The listing builds one solid part. Answer for the finished solid, in the listing's coordinates (mm). Coordinates: 2 decimals unless noted, no trailing zeros. Order: outer loops, then holes, each group sorted by start corner. A loop starts at its lowest first (then second) coordinate and runs counter-clockwise, first axis right, second up. Notation, with made-up numbers: (-33, 18.5) -> (-21, 18.5) arc R12 cw to (-21, 28.5) -> close; hole circle Ø4 at (-16, 78.25). An arc over 180 degrees is marked (long way). Answer in a Markdown table with one row per item. Add a question column.
```python
from build123d import *

# Parameters (mm, degrees)
BOSS_EXTRUDE1_DEPTH = 3


with BuildPart() as part:
    # Sketch3 → Boss-Extrude1 (new body)
    with BuildSketch(Plane.XY):
        with BuildLine():
            ThreePointArc((-21.06925633, 1.560185503), (-21.702383426, -4.120337722), (-16.861546239, -7.159332517))
            Line((-16.861546239, -7.159332517), (-16.235942246, -7.122800897))
            ThreePointArc((-16.235942246, -7.122800897), (-14.247317716, -6.480760333), (-12.653836147, -5.128850538))
            ThreePointArc((-12.653836147, -5.128850538), (21.262556938, 11.81913919), (56.062735888, -3.230898045))
            ThreePointArc((56.062735888, -3.230898045), (59.548283557, -3.823314658), (60.140700171, -0.337766989))
            ThreePointArc((60.140700171, -0.337766989), (19.96998669, 19.192613792), (-21.06925633, 1.560185503))
        make_face()
        Polygon((-14.842971244, -1.436629161), (-14.495267888, -1.784332517), (-14.848821278, -2.137885908), (-14.637840313, -2.550832882), (-15.083092963, -2.778319315), (-15.00954079, -3.236171091), (-15.503211236, -3.315477399), (-15.574237606, -3.773727796), (-16.068337858, -3.697144889), (-16.277038544, -4.111248976), (-16.723538831, -3.886221213), (-17.049626765, -4.215925369), (-17.405124343, -3.864326917), (-17.816901648, -4.077581746), (-18.046839834, -3.633590269), (-18.504279068, -3.70966601), (-18.586306367, -3.21644038), (-19.04494145, -3.147941973), (-18.971084274, -2.65342694), (-19.386332882, -2.447012878), (-19.163770631, -1.999278532), (-19.495267888, -1.67501361), (-19.145635065, -1.317582653), (-19.361157273, -0.906987537), (-18.918440472, -0.674604591), (-18.997037466, -0.217591808), (-18.504271649, -0.132846012), (-18.438303288, 0.326159812), (-17.94338851, 0.255030612), (-17.73926735, 0.671411115), (-17.290312559, 0.451321143), (-16.967880508, 0.784601421), (-16.60852704, 0.436944858), (-16.199126599, 0.654727893), (-15.964305958, 0.213299227), (-15.507733522, 0.294415085), (-15.420271807, -0.197875935), (-14.960909199, -0.261312244), (-15.029308259, -0.756611718), (-14.611808522, -0.958433771), align=None, mode=Mode.SUBTRACT)
    extrude(amount=BOSS_EXTRUDE1_DEPTH)


solid = part.part
```
Q1. Determine the mould class of faces 1 (the face through (20.7, 11.8, 1.5)), 2 (the face through (59.503, -3.855, 1.479)), 3 (the face through (-21.74, -4.04, 1.48)), 4 (the face through (-14.273, -6.495, 1.479)) for opening direction X: +X half, -X half, draft (parallel to the pull), parting line (faces both ways), or undercut.
Q2. A cutting plane is placed at B-B (y = 17.25). Determine the outline of the cut face in (x, z), then the cut area to 3 significant figures.
Q3. Straight lines are drawn through the part: line 1 (X direction, y = 1.5, z = 2.2); line 2 (X direction, y = 8.75, z = 2.55); line 3 (Y direction, x = 52, z = 0.5). For each, find the intervals that lie inside material, in ascending order.
Q4. Given pin 1 (1.5 mm diameter, centred on y = 5, z = 2, fed in from -X); pin 2 (1.5 mm diameter, centred on x = 26, z = 2, fed in from +Y); pin 3 (1.5 mm diameter, centred on x = -0.5, z = 1, fed in from -Y), each flat-ended and moving along its own axis, determine where each tip first touches the part or whether it passes through.
Q5. A cutting plane is placed at A-A (x = -2.5). Determine the outline of the cut face in (y, z).
Returned:
| question | item | result |
|---|---|---|
| 1 | face 1 | undercut |
| 1 | face 2 | undercut |
| 1 | face 3 | -X half |
| 1 | face 4 | +X half |
| 2 | outline | (4.35, 0) -> (33.08, 0) -> (33.08, 3) -> (4.35, 3) -> close |
| 2 | area | 86.2 mm² |
| 3 | line 1 | x = -21.12 to -6.16, 51.17 to 58.56 |
| 3 | line 2 | x = -13.11 to 6.14, 38.86 to 50.55 |
| 3 | line 3 | y = 0.79 to 7.64 |
| 4 | pin 1 | stops at x = -18.46 |
| 4 | pin 2 | stops at y = 18.81 |
| 4 | pin 3 | stops at y = 5.04 |
| 5 | outline | (4.23, 0) -> (14.84, 0) -> (14.84, 3) -> (4.23, 3) -> close |
